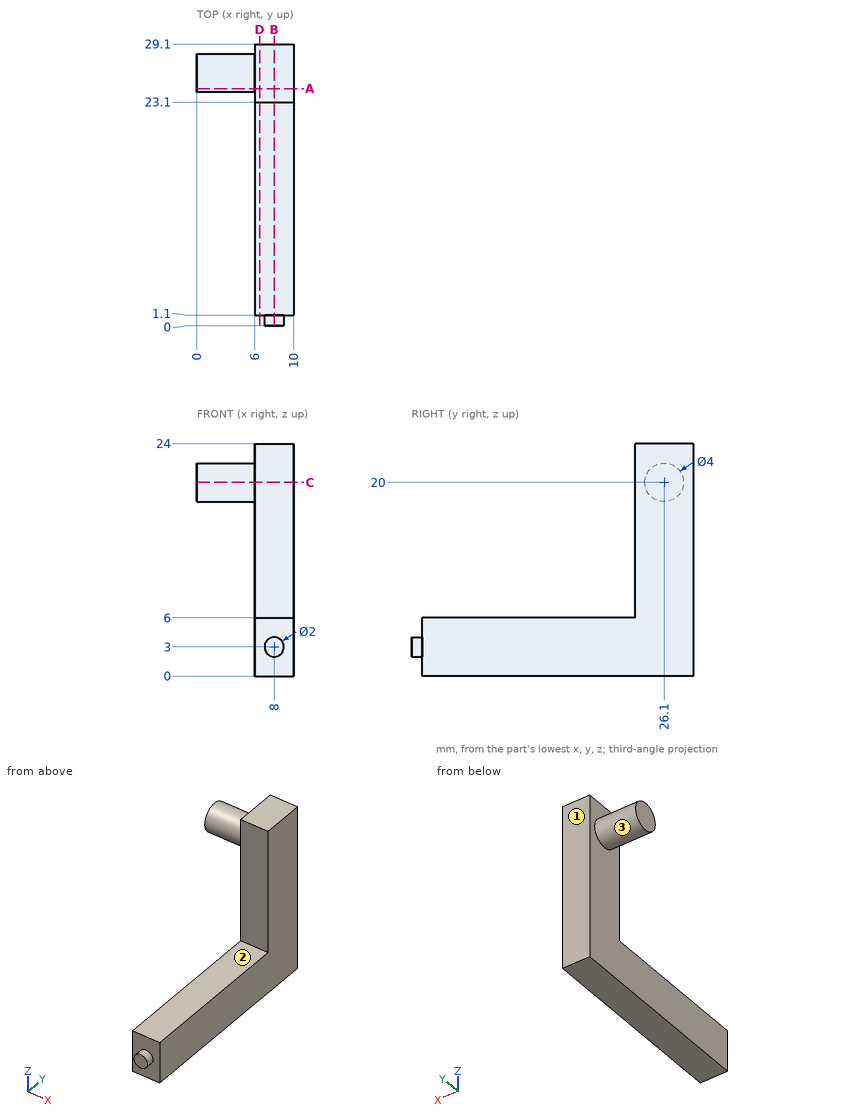
Check sheet for the drawn part. Datum: minimum x, y, z corner. Units: mm. A direction names the side the tool comes from. Coordinates: 2 decimals unless noted, no trailing zeros. Loops run counter-clockwise (first coordinate to the right, second up) from the corner with the lowest first, then second, coordinate; pieces in that order, holes last. Notation, with made-up numbers: (12.25, 7.25) - (20.25, 7.25) arc R21 cw to (20.25, 31.25) - close; hole circle Ø11 at (46.25, 3.5). An arc over 180 degrees is marked (long way). Put each result on its own line as item: value.
Item 1: Set-up check for the marked faces 1, 2 and 3: record each of +Z, -Z, +X, -X, +Y, -Y from which the full face is reachable in a straight line by a thin tool's end or side.
Conclusion:
face 1: +Z, -Z, +X, -X, +Y
face 2: +Z, +X, -X, -Y
face 3: -X
Item 2: Section check D-D (x = 6.5). Enter the section's corners in (y, z), then the cut area to 3 significant figures.
Conclusion:
outline: (1.1, 0) - (29.1, 0) - (29.1, 24) - (23.1, 24) - (23.1, 6) - (1.1, 6) - close
area: 276 mm2
Item 3: Scan lines: line 1 along Y through (x, z) = (7.75, 4); line 2 along Z through (x, y) = (9.5, 7); line 3 along X through (y, z) = (22, 3.5). Record each from-to range of solid material in increasing order.
Conclusion:
line 1: y = 1.1 to 29.1
line 2: z = 0 to 6
line 3: x = 6 to 10
Item 4: Gauge pin test, flat ends, axial feed: pin 1 Ø4 at (x, z) = (6, 6) entering from -Y; pin 2 Ø1 at (x, z) = (7, 20.5) entering from -Y; pin 3 Ø3 at (x, y) = (7.5, 8.5) entering from +Z. Record the tip position at first contact, or that the pin passes through.
Conclusion:
pin 1: stops at y = 1.1
pin 2: stops at y = 23.1
pin 3: stops at z = 6
Item 5: Section check B-B (x = 8). Enter the section's corners in (y, z).
Conclusion:
outline: (0, 2) - (1.1, 2) - (1.1, 0) - (29.1, 0) - (29.1, 24) - (23.1, 24) - (23.1, 6) - (1.1, 6) - (1.1, 4) - (0, 4) - close
Item 6: Section check C-C (z = 20). Enter the section's corners in (x, y).
Conclusion:
outline: (0, 24.1) - (6, 24.1) - (6, 23.1) - (10, 23.1) - (10, 29.1) - (6, 29.1) - (6, 28.1) - (0, 28.1) - close
Item 7: Section check A-A (y = 24.5). Enter the section's corners in (x, z), then the cut area to 3 significant figures.
Conclusion:
outline: (0, 18.8) - (6, 18.8) - (6, 0) - (10, 0) - (10, 24) - (6, 24) - (6, 21.2) - (0, 21.2) - close
area: 110 mm2
